Check sheet for the modelled part. Datum: model origin and axes. Units: mm. Face numbers are marked on the shaded views. A direction names the side the tool comes from. Give positions to 0.01 mm unless a question says otherwise; leave off trailing zeros. Order: outer loops, then holes, each group sorted by start corner. A loop starts at its lowest first (then second) coordinate and runs counter-clockwise, first axis right, second up. Notation, with made-up numbers: (68.5, 2) -> (75.5, 2) arc R10 ccw to (75.5, 15) -> close; hole circle Ø9 at (-18, 47.5). An arc over 180 degrees is marked (long way). One line per question, with ' | ' between items.
Autodesk Inventor part; units mm, degrees
ref_plane "YZ Plane" through (0, 0, 0) normal (1, 0, 0) x (0, 1, 0)
ref_plane "XZ Plane" through (0, 0, 0) normal (0, 1, 0) x (-1, 0, 0)
ref_plane "XY Plane" through (0, 0, 0) normal (0, 0, 1) x (1, 0, 0)
sketch "Sketch1" plane through (0, 0, 0) normal (1, 0, 0) x (0, 1, 0)
  line L0 (8.7098, 9.3403) -> (-28.2902, 9.3403)
  line L1 (-28.2902, 9.3403) -> (-28.2902, -31.5597)
  line L2 (-28.2902, -31.5597) -> (8.7098, -31.5597)
  line L3 (8.7098, -31.5597) -> (8.7098, 9.3403)
  line L4 (8.7098, -29.3092) -> (14.4098, -29.3092)
  line L5 (14.4098, -29.3092) -> (14.4098, -17.8188)
  line L6 (14.4098, -17.8188) -> (8.7098, -17.8188)
  line L7 (8.7098, -17.8188) -> (8.7098, -29.3092)
  point P0 (0, 0)
  dimension "d0" = 37
  dimension "d1" = 40.9
  dimension "d2" = 5.7
extrude "Extrusion1" add sketch "Sketch1" along normal blind 20
sketch "Sketch2" plane through (20, 0, 0) normal (1, 0, 0) x (0, 0, -1)
  line L0 (29.3092, 14.4098) -> (17.8188, 14.4098)
  line L1 (29.3092, 8.7098) -> (29.3092, 14.4098)
  line L2 (17.8188, 14.4098) -> (29.3092, 14.4098)
  line L3 (29.3092, 14.4098) -> (29.3092, 8.7098)
  line L4 (29.3092, 8.7098) -> (17.8188, 8.7098)
  line L5 (17.8188, 8.7098) -> (17.8188, 14.4098)
  point P0 (0, 0)
extrude "Extrusion2" cut sketch "Sketch2" against normal blind 5
sketch "Sketch3" plane through (0, 0, 0) normal (-1, 0, 0) x (0, 0, 1)
  line L0 (-17.8188, 14.4098) -> (-29.3092, 14.4098)
  line L1 (-17.8188, 8.7098) -> (-17.8188, 14.4098)
  line L2 (-29.3092, 14.4098) -> (-17.8188, 14.4098)
  line L3 (-17.8188, 14.4098) -> (-17.8188, 8.7098)
  line L4 (-17.8188, 8.7098) -> (-29.3092, 8.7098)
  line L5 (-29.3092, 8.7098) -> (-29.3092, 14.4098)
  point P0 (0, 0)
extrude "Extrusion3" cut sketch "Sketch3" against normal blind 5
sketch "Sketch4" plane through (0, 0, 0) normal (-1, 0, 0) x (0, 0, 1)
  line L0 (9.3403, -28.2902) -> (-31.5597, -28.2902)
  line L1 (9.3403, -28.2902) -> (9.3403, -1.3902)
  line L2 (9.3403, 8.7098) -> (9.3403, -28.2902)
  line L3 (9.3403, -1.3902) -> (16.8403, -1.3902)
  line L4 (16.8403, -1.3902) -> (16.8403, 1.1098)
  line L5 (16.8403, 1.1098) -> (9.3403, 1.1098)
  line L6 (9.3403, 1.1098) -> (9.3403, -1.3902)
  line L7 (-31.5597, -28.2902) -> (-31.5597, 8.7098)
  line L8 (-31.5597, -1.3902) -> (-39.0597, -1.3902)
  line L9 (-39.0597, -1.3902) -> (-39.0597, 1.1098)
  line L10 (-39.0597, 1.1098) -> (-31.5597, 1.1098)
  line L11 (-31.5597, 1.1098) -> (-31.5597, -1.3902)
  point P0 (0, 0)
  dimension "d9" = 26.9
  dimension "d10" = 7.5
  dimension "d11" = 2.5
  dimension "d12" = 7.5
extrude "Extrusion4" add sketch "Sketch4" against normal blind 20
properties part number "servo"
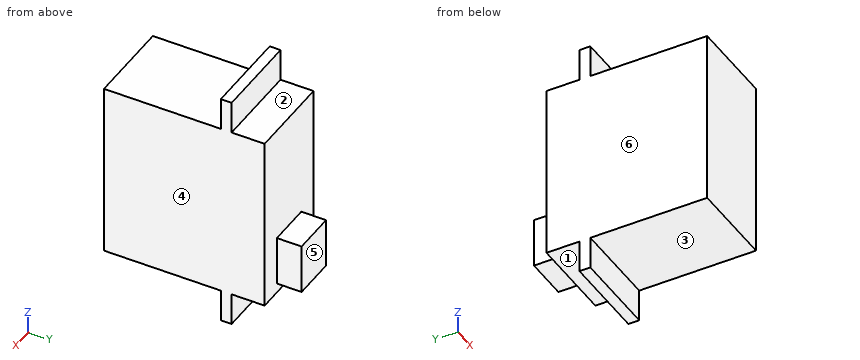
Q1. Section check A-A (x = 6.5). Enter the section's corners in (y, z), and give its area (3 significant figures).
Result sheet:
outline: (-28.29, -31.56) -> (-1.39, -31.56) -> (-1.39, -39.06) -> (1.11, -39.06) -> (1.11, -31.56) -> (8.71, -31.56) -> (8.71, -29.31) -> (14.41, -29.31) -> (14.41, -17.82) -> (8.71, -17.82) -> (8.71, 9.34) -> (1.11, 9.34) -> (1.11, 16.84) -> (-1.39, 16.84) -> (-1.39, 9.34) -> (-28.29, 9.34) -> close | area: 1,620 mm2
Q2. Section check C-C (x = 3.75). Enter the section's corners in (y, z), and give its area (3 significant figures).
Result sheet:
outline: (-28.29, -31.56) -> (-1.39, -31.56) -> (-1.39, -39.06) -> (1.11, -39.06) -> (1.11, -31.56) -> (8.71, -31.56) -> (8.71, 9.34) -> (1.11, 9.34) -> (1.11, 16.84) -> (-1.39, 16.84) -> (-1.39, 9.34) -> (-28.29, 9.34) -> close | area: 1,550 mm2
Q3. Thickness scan on line 1 (Y direction, x = 6.5, z = -16); line 2 (Y direction, x = 4, z = 10); line 3 (Z direction, x = 10.5, y = -8.5). Record the ranges inside material, lowest first.
Result sheet:
line 1: y = -28.29 to 8.71 | line 2: y = -1.39 to 1.11 | line 3: z = -31.56 to 9.34
Q4. Mould release check, pull along X, two halves, no side actions. Record for the marked faces 4, 5 and 6: pulls with the +X half, pulls with the -X half, needs draft (parallel to the pull), parting line crosses it, or undercut.
Result sheet:
face 4: pulls with the +X half | face 5: needs draft | face 6: pulls with the -X half
Q5. Section check D-D (y = -12.5). Enter the section's corners in (x, z), and give its area (3 significant figures).
Result sheet:
outline: (0, -31.56) -> (20, -31.56) -> (20, 9.34) -> (0, 9.34) -> close | area: 818 mm2
Q6. Section check B-B (z = -26.5). Enter the section's corners in (x, y).
Result sheet:
outline: (0, -28.29) -> (20, -28.29) -> (20, 8.71) -> (15, 8.71) -> (15, 14.41) -> (5, 14.41) -> (5, 8.71) -> (0, 8.71) -> close
Q7. Access from +Z, -Z, +X, -X, +Y, -Y to the whole of each face (thin tool, end or side, straight path). Record for the marked faces 1, 2 and 3.
Result sheet:
face 1: -Z, +X, -X, +Y | face 2: +Z, +X, -X, +Y | face 3: -Z, +X, -X, -Y
Q8. Depth check by flat-ended pin: pin 1 Ø4.5 at (y, z) = (11, -20.5) entering from -X; pin 2 Ø10 at (x, y) = (7, -12) entering from +Z; pin 3 Ø8 at (x, z) = (10, 13.5) entering from -Y. Enter the tip coordinate at first touch or a pass-through.
Result sheet:
pin 1: stops at x = 5 | pin 2: stops at z = 9.34 | pin 3: stops at y = -1.39
